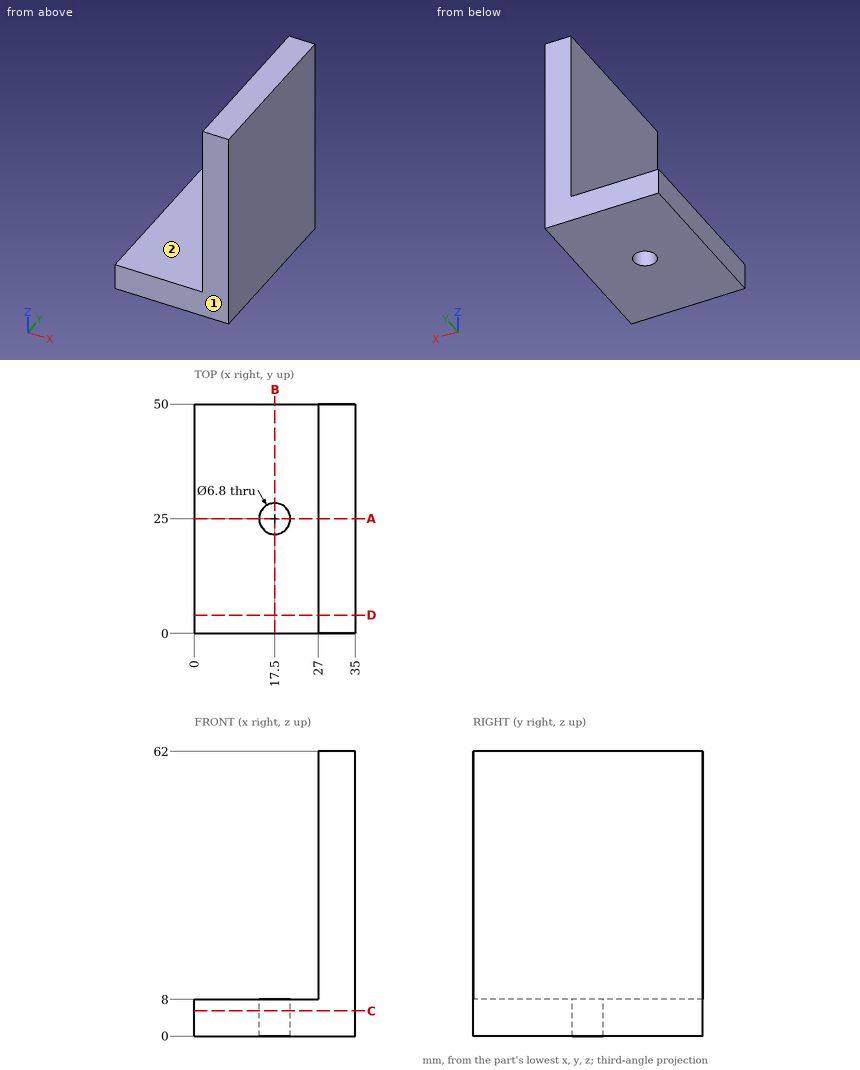
Study the drawing (mm; zero at the part's minimum x, y, z) and answer. A direction names the side the tool comes from. Give positions to 0.01 mm unless a question says otherwise; leave off trailing zeros. Order: outer loops, then holes, each group sorted by start corner. A loop starts at its lowest first (then second) coordinate and runs counter-clockwise, first axis right, second up. Notation, with made-up numbers: (87.25, 84) - (139.25, 84) arc R26 ccw to (139.25, 104) - close; hole circle Ø1 at (-10.75, 74). An arc over 180 degrees is marked (long way). Answer in a Markdown table with one row per item. Add a question column.
Q1. Find the intervals of material crossed by line 1 along X through (y, z) = (25, 5.75); line 2 along Y through (x, z) = (17.5, 2.5); line 3 along Z through (x, y) = (10, 28.5), in increasing order. Write a range as [from, to].
Q2. The part is cut by section A-A (y = 25). Determine the outline of the cut face in (x, z), then the cut area to 3 significant figures.
Q3. The part is cut by section B-B (x = 17.5). Determine the outline of the cut face in (y, z), then the cut area to 3 significant figures.
Q4. The part is cut by section C-C (z = 5.5). Determine the outline of the cut face in (x, y).
Q5. The part is cut by section D-D (y = 4). Determine the outline of the cut face in (x, z), then the cut area to 3 significant figures.
Q6. Which of the six approach directions +Z, -Z, +X, -X, +Y, -Y give full straight-line access (tool end or side, diameter ignored) to the marked faces 1 and 2?
Q7. Given P1, Ø10, axis at y = 36.5, z = 34.5, coming from the -X side; P2, Ø11, axis at x = 17.5, y = 25, coming from the +Z side; P3, Ø4, axis at x = 18, y = 23, coming from the -Z side, each flat-ended and moving along its own axis, determine where each tip first touches the part or whether it passes through.
Determined:
| question | item | result |
|---|---|---|
| 1 | line 1 | x = [0, 14.1], [20.9, 35] |
| 1 | line 2 | y = [0, 21.6], [28.4, 50] |
| 1 | line 3 | z = [0, 8] |
| 2 | outline | (0, 0) - (14.1, 0) - (14.1, 8) - (0, 8) - close; (20.9, 0) - (35, 0) - (35, 62) - (27, 62) - (27, 8) - (20.9, 8) - close |
| 2 | area | 658 mm² |
| 3 | outline | (0, 0) - (21.6, 0) - (21.6, 8) - (0, 8) - close; (28.4, 0) - (50, 0) - (50, 8) - (28.4, 8) - close |
| 3 | area | 346 mm² |
| 4 | outline | (0, 0) - (35, 0) - (35, 50) - (0, 50) - close; hole circle Ø6.8 at (17.5, 25) |
| 5 | outline | (0, 0) - (35, 0) - (35, 62) - (27, 62) - (27, 8) - (0, 8) - close |
| 5 | area | 712 mm² |
| 6 | face 1 | +Z, -Z, +X, -X, -Y |
| 6 | face 2 | +Z, -X, +Y, -Y |
| 7 | P1 | stops at x = 27 |
| 7 | P2 | stops at z = 8 |
| 7 | P3 | stops at z = 0 |
